```python
from build123d import *

# Parameters (mm, degrees)
SKETCH1_R                    = 17.4625
BOSS_EXTRUDE1_DEPTH          = 4.1275
SKETCH2_R                    = 28.575
BOSS_EXTRUDE2_DEPTH          = 3.175
F_10_0_1935_DIAMETER_HOLE1_D = 4.9149
CIRPATTERN1_COUNT            = 8
CUT_EXTRUDE1_REACH           = 43.066
SKETCH5_R                    = 9.525


with BuildPart() as part:
    # Sketch1 → Boss-Extrude1 (new body)
    with BuildSketch(Plane.XY):
        Circle(SKETCH1_R)
    extrude(amount=BOSS_EXTRUDE1_DEPTH)

    # Sketch2 → Boss-Extrude2 (add)
    with BuildSketch(Plane(origin=(0, 0, 0), x_dir=(-1, 0, 0), z_dir=(0, 0, -1))):
        Circle(SKETCH2_R)
    extrude(amount=BOSS_EXTRUDE2_DEPTH)

    # #10 (0.1935) Diameter Hole1 (through all)
    with Locations(Plane(origin=(0, 0, -3.175), x_dir=(-1, 0, 0), z_dir=(0, 0, -1))):
        with Locations((0, 22.225)):
            f_10_0_1935_diameter_hole1 = Hole(F_10_0_1935_DIAMETER_HOLE1_D / 2)

    # CirPattern1: #10 (0.1935) Diameter Hole1 ×8 about axis
    cirpattern1_axis = Axis((0, 0, 0), (0, 0, 1))
    for i in range(1, CIRPATTERN1_COUNT):
        add(f_10_0_1935_diameter_hole1.rotate(cirpattern1_axis, i * 360 / CIRPATTERN1_COUNT), mode=Mode.SUBTRACT)

    # Sketch5 → Cut-Extrude1 (cut, up to next)
    with BuildSketch(Plane(origin=(0, 0, -3.175), x_dir=(-1, 0, 0), z_dir=(0, 0, -1)), mode=Mode.PRIVATE) as cut_extrude1_sk1:
        Circle(SKETCH5_R)
    cut_extrude1_tool1 = extrude(cut_extrude1_sk1.sketch, amount=-CUT_EXTRUDE1_REACH, mode=Mode.PRIVATE) & part.part
    add(cut_extrude1_tool1.solids().sort_by_distance((0, 0, -3.175))[0], mode=Mode.SUBTRACT)


solid = part.part
```
CAD build for the part. Positions are in the model's coordinates, mm. A direction names the side the tool comes from. Round coordinates to 2 decimals unless told otherwise and drop trailing zeros. Order: outer loops, then holes, each group sorted by start corner. A loop starts at its lowest first (then second) coordinate and runs counter-clockwise, first axis right, second up.
Item 1: Saw through at A-A on x = 0. Write the cut outline in (y, z) (1 decimal), then the cut area to 3 significant figures.
Item 2: Saw through at C-C on x = 23. Write the cut outline in (y, z) (3 decimals).
Item 3: Tool access for faces 4 (the face through (-16.04, 13.28, -1.57)), 5 (the face through (-13.858, -10.626, 2.035)): list every direction of +Z, -Z, +X, -X, +Y, -Y with a clear straight run to the whole face (end or side of a thin tool).
Item 4: Mould opens along X. For faces 1 (the face through (13, -12, 0)), 2 (the face through (13.28, 16.04, -1.57)), 3 (the face through (28.547, 1.256, -1.565)) say: pulls with the +X half, pulls with the -X half, needs draft (parallel to the pull), parting line crosses it, or undercut.
Item 5: Pin check, flat tips, straight feed: pin 1 (5.5 mm diameter, centred on x = 0, y = -22.225, fed in from -Z) (3 decimals); pin 2 (1.5 mm diameter, centred on y = 5.5, z = 1, fed in from +X); pin 3 (4 mm diameter, centred on x = 0, y = 22.225, fed in from +Z); pin 4 (4 mm diameter, centred on y = 16, z = 1.5, fed in from -X). Stop position of each tip, or through.
Item 6: Probe line 1 along Y through (x, z) = (0, -2.05) (3 decimals); line 2 along Y through (x, z) = (0, 2.5) (1 decimal); line 3 along Z through (x, y) = (6.5, -19) (3 decimals). List the from-to ranges inside material, lowest first.
Item 7: Saw through at B-B on y = -4. Write the cut outline in (x, z) (1 decimal).
Reported:
1. outline: (-28.6, -3.2) - (-24.7, -3.2) - (-24.7, 0) - (-28.6, 0) - close; (-19.8, -3.2) - (-9.5, -3.2) - (-9.5, 4.1) - (-17.5, 4.1) - (-17.5, 0) - (-19.8, 0) - close; (9.5, -3.2) - (19.8, -3.2) - (19.8, 0) - (17.5, 0) - (17.5, 4.1) - (9.5, 4.1) - close; (24.7, -3.2) - (28.6, -3.2) - (28.6, 0) - (24.7, 0) - close
1. area: 155 mm2
2. outline: (-16.957, -3.175) - (-2.332, -3.175) - (-2.332, 0) - (-16.957, 0) - close; (2.332, -3.175) - (16.957, -3.175) - (16.957, 0) - (2.332, 0) - close
3. face 4: +Z, -Z
3. face 5: +Z
4. face 1: needs draft
4. face 2: undercut
4. face 3: parting line crosses it
5. pin 1: stops at z = -3.175
5. pin 2: stops at x = 16.8
5. pin 3: passes through
5. pin 4: stops at x = -24.52
6. line 1: y = -28.575 to -24.682, -19.768 to -9.525, 9.525 to 19.768, 24.682 to 28.575
6. line 2: y = -17.5 to -9.5, 9.5 to 17.5
6. line 3: z = -3.175 to 0
7. outline: (-28.3, -3.2) - (-8.6, -3.2) - (-8.6, 4.1) - (-17, 4.1) - (-17, 0) - (-28.3, 0) - close; (8.6, -3.2) - (28.3, -3.2) - (28.3, 0) - (17, 0) - (17, 4.1) - (8.6, 4.1) - close
